Autodesk Inventor part; units mm, degrees
ref_plane "YZ Plane" through (0, 0, 0) normal (1, 0, 0) x (0, 1, 0)
ref_plane "XZ Plane" through (0, 0, 0) normal (0, 1, 0) x (-1, 0, 0)
ref_plane "XY Plane" through (0, 0, 0) normal (0, 0, 1) x (1, 0, 0)
sketch "Sketch1" plane through (0, 0, 0) normal (0, 1, 0) x (-1, 0, 0)
  line L0 (36.926, 42.926) -> (-36.926, 42.926)
  line L1 (-42.926, 36.926) -> (-42.926, -36.926)
  line L2 (-36.926, -42.926) -> (36.926, -42.926)
  line L3 (42.926, -36.926) -> (42.926, 36.926)
  line L4 (55, 0) -> (-75, 0) construction
  line L5 (0, 74) -> (0, -88) construction
  arc A0 (42.926, 36.926) -> (36.926, 42.926) centre (36.926, 36.926) ccw
  arc A1 (36.926, -42.926) -> (42.926, -36.926) centre (36.926, -36.926) ccw
  arc A2 (-42.926, -36.926) -> (-36.926, -42.926) centre (-36.926, -36.926) ccw
  arc A3 (-36.926, 42.926) -> (-42.926, 36.926) centre (-36.926, 36.926) ccw
  circle A4 centre (34.798, 34.798) radius 2.7559
  circle A5 centre (34.798, -34.798) radius 2.7559
  circle A6 centre (-34.798, -34.798) radius 2.7559
  circle A7 centre (-34.798, 34.798) radius 2.7559
  point P0 (0, 0)
  point P1 (42.926, 42.926)
  point P2 (42.926, -42.926)
  point P3 (42.926, 0)
  point P4 (0, -42.926)
  dimension "d0" = 85.852
  dimension "d1" = 6
  dimension "d5" = 5.5118
  dimension "d6" = 69.596
  dimension "d7" = 69.596
  dimension "d8" = 69.596
  dimension "d9" = 69.596
  dimension "d10" = 34.798
  dimension "d11" = 34.798
extrude "Extrusion1" add sketch "Sketch1" along normal blind 8.382
sketch "Sketch2" plane through (0, 8.382, 0) normal (0, 1, 0) x (1, 0, 0)
  line L0 (42.926, -28) -> (42.926, 28)
  line L1 (-42.926, 28) -> (-42.926, -28)
  line L2 (-28, -42.926) -> (28, -42.926)
  line L3 (28, 42.926) -> (-28, 42.926)
  line L4 (-42.926, 36.926) -> (-42.926, -36.926)
  line L5 (36.926, 42.926) -> (-36.926, 42.926)
  line L6 (42.926, -36.926) -> (42.926, 36.926)
  line L7 (-36.926, -42.926) -> (36.926, -42.926)
  line L8 (-42.926, -28) -> (-33, -28)
  line L9 (33, -28) -> (42.926, -28)
  line L10 (-28, 42.926) -> (-28, 33)
  line L11 (-28, -33) -> (-28, -42.926)
  line L12 (42.926, 28) -> (33, 28)
  line L13 (-33, 28) -> (-42.926, 28)
  line L14 (28, -42.926) -> (28, -33)
  line L15 (28, 33) -> (28, 42.926)
  arc A0 (33, -28) -> (28, -33) centre (33, -33) ccw
  arc A1 (-28, -33) -> (-33, -28) centre (-33, -33) ccw
  arc A2 (-33, 28) -> (-28, 33) centre (-33, 33) ccw
  arc A3 (28, 33) -> (33, 28) centre (33, 33) ccw
  point P0 (0, 0)
  dimension "d14" = 56
  dimension "d16" = 56
  dimension "d18" = 5
  dimension "d30" = 28
  dimension "d31" = 28
extrude "Extrusion2" add sketch "Sketch2" along normal blind 80.01
fillet "Fillet1" radius 3 16 edges at (29.4645, 88.392, 29.4645) (28, 88.392, 37.963) (37.963, 88.392, 28) (42.926, 88.392, 0) (0, 88.392, -42.926) (-42.926, 88.392, 0) (-28, 88.392, 37.963) (-37.963, 88.392, 28) (-29.4645, 88.392, 29.4645) (0, 88.392, 42.926) (29.4645, 88.392, -29.4645) (28, 88.392, -37.963) (37.963, 88.392, -28) (-29.4645, 88.392, -29.4645) (-28, 88.392, -37.963) (-37.963, 88.392, -28)
sketch "Sketch3" plane through (0, 0, 0) normal (0, -1, 0) x (1, 0, 0)
  circle A0 centre (0, 0) radius 6.35
  dimension "d22" = 12.7
extrude "Extrusion3" add sketch "Sketch3" along normal blind 31.75
properties part number "1224_Stepper Motor_V1"
Part model, mm, in its own coordinate system. A direction names the side the tool comes from. Coordinates: 2 decimals unless noted, no trailing zeros. Loops run counter-clockwise (first coordinate to the right, second up) from the corner with the lowest first, then second, coordinate; pieces in that order, holes last. Notation, with made-up numbers: (31.25, 82.5) - (75.25, 82.5) arc R21 ccw to (75.25, 94.5) - close; hole circle Ø4 at (20, -17.5). An arc over 180 degrees is marked (long way). Write item = value, one per line. Start each with the question number.
Item 1: Cut at A-A, the plane y = 17.5. Give the cut face in (x, z), and give its area (3 significant figures).
Item 2: Cut at C-C, the plane x = 0. Give the cut face in (y, z), and give its area (3 significant figures).
Item 3: Wall check: L1, parallel to Y at x = 31, z = 16; L2, parallel to Z at x = 35.5, y = 18; L3, parallel to Y at x = -38, z = 34. Give the ranges that are in metal, low to high. Write a range as from..to.
Item 4: Flat gauge pins, fed straight in: pin 1 Ø3 at (x, y) = (-33.5, 69.5) entering from -Z; pin 2 Ø2 at (x, z) = (3.5, -34) entering from -Y; pin 3 Ø5 at (x, y) = (-37.5, 29) entering from +Z. Where does each tip first touch, or does it go through?
Item 5: Mould opens along X. For faces 1 (the cylindrical face through (-34.2, 4.13, 37.49)), 2 (the flat face through (-28, 46, 38)), 3 (the cylindrical face through (30, 46, -29)) say: released by +X, released by -X, zero draft, split by the parting line, or undercut.
Item 6: Cut at B-B, the plane z = 0. Give the cut face in (x, y).
Item 7: Cut at D-D, the plane z = 14. Give the cut face in (x, y), and give its area (3 significant figures).
Item 8: 3-axis set-ups, long thin cutter, end or side, ignore diameter. For faces 4 (the flat face through (-37, 8.382, 37)), 5 (the flat face through (-38, 46, -28)), 6 (the flat face through (37, 8.382, 37)), 7 (the cylindrical face through (38.032, 87.49, -27.145)): which of +Z, -Z, +X, -X, +Y, -Y reach the whole face in a straight line?
The answers:
q1.outline = (-42.93, -28) - (-33, -28) arc R5 cw to (-28, -33) - (-28, -42.93) - (28, -42.93) - (28, -33) arc R5 cw to (33, -28) - (42.93, -28) - (42.93, 28) - (33, 28) arc R5 cw to (28, 33) - (28, 42.93) - (-28, 42.93) - (-28, 33) arc R5 cw to (-33, 28) - (-42.93, 28) - close
q1.area = 6,500 mm2
q2.outline = (-31.75, -6.35) - (0, -6.35) - (0, -42.93) - (85.39, -42.93) arc R3 ccw to (88.39, -39.93) - (88.39, 39.93) arc R3 ccw to (85.39, 42.93) - (0, 42.93) - (0, 6.35) - (-31.75, 6.35) - close
q2.area = 7,990 mm2
q3.L1 = 0..88.39
q3.L2 = -28..28
q3.L3 = 0..8.38
q4.pin_1 = -28.1
q4.pin_2 = 0
q4.pin_3 = 28
q5.face_1 = undercut
q5.face_2 = released by -X
q5.face_3 = released by +X
q6.outline = (-42.93, 0) - (-6.35, 0) - (-6.35, -31.75) - (6.35, -31.75) - (6.35, 0) - (42.93, 0) - (42.93, 85.39) arc R3 ccw to (39.93, 88.39) - (-39.93, 88.39) arc R3 ccw to (-42.93, 85.39) - close
q7.outline = (-42.93, 0) - (42.93, 0) - (42.93, 85.39) arc R3 ccw to (39.93, 88.39) - (-39.93, 88.39) arc R3 ccw to (-42.93, 85.39) - close
q7.area = 7,580 mm2
q8.face_4 = +Z, -X, +Y
q8.face_5 = -Z, -X, +Y
q8.face_6 = +Z, +X, +Y
q8.face_7 = -Z, +X, +Y
